from build123d import *

# Parameters (mm, degrees)
SKETCH2_W           = 160
SKETCH2_H           = 28.45
BOSS_EXTRUDE1_DEPTH = 10
SKETCH4_W           = 60
SKETCH4_H           = 10
BOSS_EXTRUDE2_DEPTH = 5
SKETCH5_R           = 2.5
CUT_EXTRUDE1_DEPTH  = 83.883053907
BOSS_EXTRUDE3_DEPTH = 1


with BuildPart() as part:
    # Sketch2 → Boss-Extrude1 (new body)
    with BuildSketch(Plane(origin=(0, 0, 0), x_dir=(1, 0, 0), z_dir=(0, 1, 0))):
        Rectangle(SKETCH2_W, SKETCH2_H)
    extrude(amount=BOSS_EXTRUDE1_DEPTH)

    # Sketch4 → Boss-Extrude2 (add)
    with BuildSketch(Plane.XY.offset(14.225)):
        with Locations((0, 5)):
            Rectangle(SKETCH4_W, SKETCH4_H)
    extrude(amount=BOSS_EXTRUDE2_DEPTH)

    # Sketch5 → Cut-Extrude1 (cut, through all)
    with BuildSketch(Plane(origin=(0, 10, 0), x_dir=(1, 0, 0), z_dir=(0, 1, 0))):
        with Locations(Location((70, -6.225, 0), (0, 0, 270))):
            Circle(SKETCH5_R)
        with Locations(Location((30, -6.225, 0), (0, 0, 270))):
            Circle(SKETCH5_R)
        with Locations(Location((-30, -6.225, 0), (0, 0, 90))):
            Circle(SKETCH5_R)
        with Locations(Location((-70, -6.225, 0), (0, 0, 90))):
            Circle(SKETCH5_R)
    extrude(amount=-CUT_EXTRUDE1_DEPTH, mode=Mode.SUBTRACT)

    # Sketch6 → Boss-Extrude3 (add)
    with BuildSketch(Plane(origin=(0, 10, 0), x_dir=(1, 0, 0), z_dir=(0, 1, 0))):
        Polygon((3.95, 14.225), (3.95, 7.725), (7, 7.725), (7, 1.225), (0, 1.225), (-7, 1.225), (-7, 7.725), (-3.95, 7.725), (-3.95, 14.225), align=None)
        Polygon((-17.95, 14.225), (-25.85, 14.225), (-25.85, 7.725), (-28.9, 7.725), (-28.9, 1.225), (-21.9, 1.225), (-14.9, 1.225), (-14.9, 7.725), (-17.95, 7.725), align=None)
        Polygon((-39.85, 14.225), (-47.75, 14.225), (-47.75, 7.725), (-50.8, 7.725), (-50.8, 1.225), (-43.8, 1.225), (-36.8, 1.225), (-36.8, 7.725), (-39.85, 7.725), align=None)
        Polygon((-61.75, 14.225), (-69.65, 14.225), (-69.65, 7.725), (-72.7, 7.725), (-72.7, 1.225), (-65.7, 1.225), (-58.7, 1.225), (-58.7, 7.725), (-61.75, 7.725), align=None)
        Polygon((25.85, 14.225), (17.95, 14.225), (17.95, 7.725), (14.9, 7.725), (14.9, 1.225), (21.9, 1.225), (28.9, 1.225), (28.9, 7.725), (25.85, 7.725), align=None)
        Polygon((47.75, 14.225), (39.85, 14.225), (39.85, 7.725), (36.8, 7.725), (36.8, 1.225), (43.8, 1.225), (50.8, 1.225), (50.8, 7.725), (47.75, 7.725), align=None)
        Polygon((69.65, 14.225), (61.75, 14.225), (61.75, 7.725), (58.7, 7.725), (58.7, 1.225), (65.7, 1.225), (72.7, 1.225), (72.7, 7.725), (69.65, 7.725), align=None)
    extrude(amount=BOSS_EXTRUDE3_DEPTH)


solid = part.part
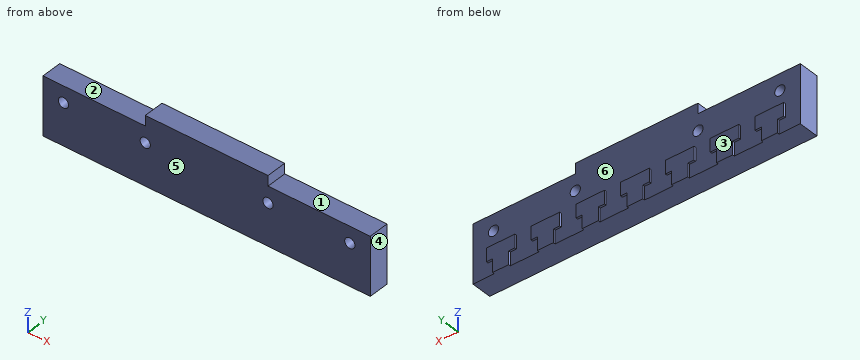
Read the model definition and answer for the solid it produces. Units are mm, in the model's axes. Face numbers are marked on the shaded views. A direction names the side the tool comes from. Round coordinates to 2 decimals unless told otherwise and drop trailing zeros. Write each loop counter-clockwise with the first axis right and the second up, starting at its lowest first coordinate (ties: lowest second). Pieces come first, ordered by that corner, then holes.
1. The part is cut by section B-B, the plane x = -38.5. Determine the outline of the cut face in (y, z) (3 decimals), then the cut area to 3 significant figures.
2. The part is cut by section A-A, the plane y = 4.5. Determine the outline of the cut face in (x, z) (3 decimals), then the cut area to 3 significant figures.
3. The part is cut by section D-D, the plane x = 55. Determine the outline of the cut face in (y, z) (3 decimals).
4. Given pin 1 Ø0.5 at (y, z) = (10.5, -11) entering from -X; pin 2 Ø1 at (x, y) = (37, 1.5) entering from +Z (3 decimals); pin 3 Ø0.5 at (x, y) = (-27.5, 10.5) entering from -Z (3 decimals); pin 4 Ø4.5 at (x, z) = (70, 6.225) entering from +Y, each flat-ended and moving along its own axis, determine where each tip first touches the part or whether it passes through.
5. The part is cut by section C-C, the plane z = 5.5. Determine the outline of the cut face in (x, y), then the cut area to 3 significant figures.
6. Determine the mould class of the marked faces 4, 5 and 6 for opening direction X: pulls with the +X half, pulls with the -X half, needs draft (parallel to the pull), parting line crosses it, or undercut.
7. Straight lines are drawn through the part: L1, parallel to X at y = 8.25, z = 6.5; L2, parallel to Y at x = 5.5, z = 6; L3, parallel to X at y = 7, z = 5. For each, find the intervals that lie inside material, in ascending order.
8. Which of the six approach directions +Z, -Z, +X, -X, +Y, -Y give full straight-line access (tool end or side, diameter ignored) to the marked faces 1, 2 and 3?
Values:
1. outline: (0, -14.225) - (10, -14.225) - (10, -7.725) - (11, -7.725) - (11, -1.225) - (10, -1.225) - (10, 14.225) - (0, 14.225) - close
1. area: 291 mm2
2. outline: (-80, -14.225) - (80, -14.225) - (80, 14.225) - (30, 14.225) - (30, 19.225) - (-30, 19.225) - (-30, 14.225) - (-80, 14.225) - close; hole circle Ø5 at (-70, 6.225); hole circle Ø5 at (-30, 6.225); hole circle Ø5 at (30, 6.225); hole circle Ø5 at (70, 6.225)
2. area: 4,770 mm2
3. outline: (0, -14.225) - (10, -14.225) - (10, 14.225) - (0, 14.225) - close
4. pin 1: stops at x = -69.65
4. pin 2: stops at z = 14.225
4. pin 3: stops at z = -7.725
4. pin 4: passes through
5. outline: (-80, 0) - (-72.39, 0) - (-72.39, 10) - (-80, 10) - close; (-67.61, 0) - (-32.39, 0) - (-32.39, 10) - (-67.61, 10) - close; (-27.61, 0) - (27.61, 0) - (27.61, 10) - (-27.61, 10) - close; (32.39, 0) - (67.61, 0) - (67.61, 10) - (32.39, 10) - close; (72.39, 0) - (80, 0) - (80, 10) - (72.39, 10) - close
5. area: 1,410 mm2
6. face 4: pulls with the +X half
6. face 5: needs draft
6. face 6: undercut
7. L1: x = -80 to -72.48, -67.52 to -32.48, -27.52 to 27.52, 32.48 to 67.52, 72.48 to 80
7. L2: y = 0 to 10
7. L3: x = -80 to -72.18, -67.82 to -32.18, -27.82 to 27.82, 32.18 to 67.82, 72.18 to 80
8. face 1: +Z, +X, +Y, -Y
8. face 2: +Z, -X, +Y, -Y
8. face 3: +Z, -Z, +X, -X, +Y
